Design review of the part built by this model. Coordinates are the model's own, in mm. Coordinates: 2 decimals unless noted, no trailing zeros. Write each loop counter-clockwise with the first axis right and the second up, starting at its lowest first coordinate (ties: lowest second). Pieces come first, ordered by that corner, then holes. Notation, with made-up numbers: M 79.25,76 L 83.25,76 A30 ccw 83.25,108 Z; hole C -36,72.5 d8. An arc over 180 degrees is marked long. Write item = value, one per line.
```python
from build123d import *

# Parameters (mm, degrees)
EXTRUDE_1_DEPTH     = 76
SKETCH_2_R          = 1.55
CUT_EXTRUDE_1_DEPTH = 79.390050389
FILLET_1_R          = 2
SKETCH_3_R          = 2.75
CUT_EXTRUDE_2_DEPTH = 8


with BuildPart() as part:
    # 草图1 → 凸台-拉伸1 (new body)
    with BuildSketch(Plane.XY):
        Polygon((0, 0), (15, 0), (9.404308102, 12), (2.115923769, 12), align=None)
    extrude(amount=EXTRUDE_1_DEPTH)

    # 草图2 → 切除-拉伸1 (cut, through all)
    with BuildSketch(Plane.XZ):
        with Locations(Location((6, 63, 0), (0, 0, 270))):
            Circle(SKETCH_2_R)
        with Locations(Location((6, 13, 0), (0, 0, 270))):
            Circle(SKETCH_2_R)
        with Locations(Location((6, 38, 0), (0, 0, 270))):
            Circle(SKETCH_2_R)
    extrude(amount=-CUT_EXTRUDE_1_DEPTH, mode=Mode.SUBTRACT)

    # 圆角1
    fillet_1_edges = [part.edges().sort_by_distance(p)[0] for p in [
        (12.202154051, 6, 76),
        (5.760115935, 12, 76),
        (1.057961884, 6, 76),
        (5.760115935, 12, 0),
        (12.202154051, 6, 0),
        (7.5, 0, 0),
        (1.057961884, 6, 0),
        (2.115923769, 12, 38),
        (9.404308102, 12, 38),
        (15, 0, 38),
        (0, 0, 38),
        (7.5, 0, 76),
    ]]
    fillet(fillet_1_edges, radius=FILLET_1_R)

    # 草图3 → 切除-拉伸2 (cut)
    with BuildSketch(Plane(origin=(0, 12, 0), x_dir=(1, 0, 0), z_dir=(0, 1, 0))):
        with Locations(Location((6, -13, 0), (0, 0, 270))):
            Circle(SKETCH_3_R)
        with Locations(Location((6, -38, 0), (0, 0, 270))):
            Circle(SKETCH_3_R)
        with Locations(Location((6, -63, 0), (0, 0, 270))):
            Circle(SKETCH_3_R)
    extrude(amount=-CUT_EXTRUDE_2_DEPTH, mode=Mode.SUBTRACT)


solid = part.part
```
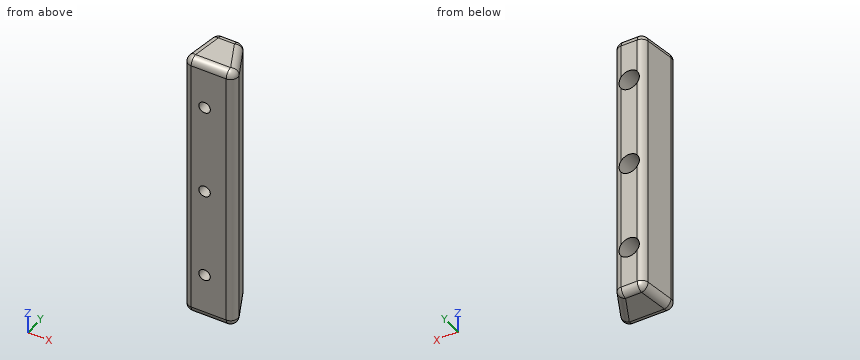
Q1. Consider section A-A, the plane x = 6. State how many separate pieces and enclosed holes the cut face has, and give its area (3 significant figures).
Check result:
separate_pieces = 4
enclosed_holes = 0
area = 739 mm²
Q2. Consider section C-C, the plane z = 38. State the section outline as (x, y) points, and give its area (3 significant figures).
Check result:
outline = M 0.41,2.35 A2 ccw 2.38,0 L 4.45,0 L 4.45,4 L 3.25,4 L 3.25,11.92 A2 ccw 1.82,10.35 Z; M 7.55,0 L 11.86,0 A2 ccw 13.67,2.85 L 9.94,10.85 A2 ccw 8.75,11.9 L 8.75,4 L 7.55,4 Z
area = 73.0 mm²
Q3. Consider section B-B, the plane z = 20. State the section outline as (x, y) points.
Check result:
outline = M 0.41,2.35 A2 ccw 2.38,0 L 11.86,0 A2 ccw 13.67,2.85 L 9.94,10.85 A2 ccw 8.13,12 L 3.79,12 A2 ccw 1.82,10.35 Z
Q4. Wall thickness on line 1 (Z direction, x = 6, y = 10); line 2 (Z direction, x = 3.75, y = 4.5); line 3 (X direction, y = 7.5, z = 13): over which ranges is each line inside the solid? List them lowest first.
Check result:
line_1 = 0 to 10.25, 15.75 to 35.25, 40.75 to 60.25, 65.75 to 76
line_2 = 0 to 11.42, 14.58 to 36.42, 39.58 to 61.42, 64.58 to 76
line_3 = 1.32 to 3.25, 8.75 to 11.5
Q5. For P1, Ø6, axis at y = 7, z = 46.5, coming from the -X side; P2, Ø1.9, axis at x = 6, z = 38, coming from the -Y side, all flat-tipped, find the tip position at first contact; note any pin that passes through.
Check result:
P1 = 0.71
P2 = through
